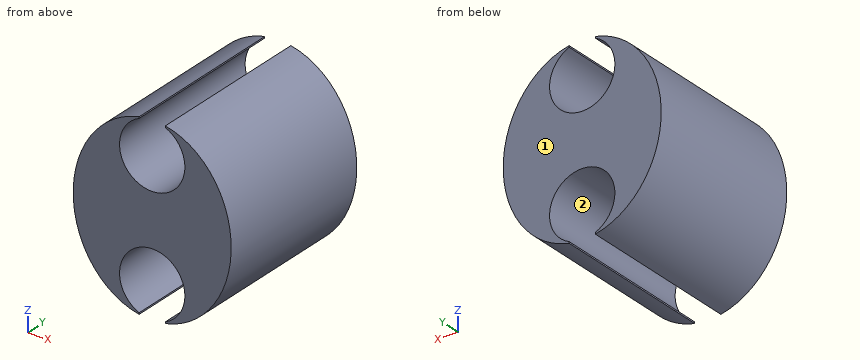
Autodesk Inventor part; units mm, degrees
ref_plane "YZ Plane" through (0, 0, 0) normal (1, 0, 0) x (0, 1, 0)
ref_plane "XZ Plane" through (0, 0, 0) normal (0, 1, 0) x (-1, 0, 0)
ref_plane "XY Plane" through (0, 0, 0) normal (0, 0, 1) x (1, 0, 0)
sketch "Boceto1" plane through (0, 0, 0) normal (0, 1, 0) x (-1, 0, 0)
  ellipse E0 centre (0, 0) end of major axis (0, 7) minor radius 6.05
  circle A0 centre (0, -4.5) radius 2.5
  circle A1 centre (0, 4.5) radius 2.5
  point P0 (0, 7)
  point P1 (0, -7)
  dimension "d0" = 7
  dimension "d1" = 6.05
  dimension "d6" = 5
  dimension "d7" = 5
extrude "Extrusión1" add sketch "Boceto1" along normal blind 13
sketch "Boceto2" plane through (0, 13, 4.5) normal (0, 1, 0) x (1, 0, 0)
  line L0 (-1, -2) -> (1, -2)
  line L1 (1, -2) -> (1, -4)
  line L2 (1, -4) -> (-1, -4)
  line L3 (-1, -4) -> (-1, -2)
  circle A0 centre (0, 0) radius 2.5
  point P0 (0, 4.5)
  point P1 (0, -2.5)
  dimension "d8" = 2
  dimension "d9" = 1
  dimension "d11" = 2
  dimension "d12" = 2
extrude "Extrusión2" cut sketch "Boceto2" against normal blind 13 contours L0 L1 A0 L3 | A0 L1 L2 L3 picked at (0, -2.1667)
sketch "Boceto4" plane through (0, 13, 0) normal (0, 1, 0) x (1, 0, 0)
  line L0 (-1, 8) -> (1, 8)
  line L1 (1, 8) -> (1, 4.3137)
  line L2 (1, 4.3137) -> (-1, 4.3137)
  line L3 (-1, 4.3137) -> (-1, 8)
  point P0 (0, 0)
  dimension "d15" = 2
  dimension "d16" = 4.3137
  dimension "d17" = 8
  dimension "d18" = 1
extrude "Extrusión3" cut sketch "Boceto4" against normal blind 13
equation "\"d7\" = d6"
properties part number "Relleno_chumacera" material "Plástico PC/ABS"
Geometry: final body of the model. Coordinates: model frame, mm. Face numbers are marked on the shaded views. Coordinates: 2 decimals unless noted, no trailing zeros. Order: outer loops, then holes, each group sorted by start corner. A loop starts at its lowest first (then second) coordinate and runs counter-clockwise, first axis right, second up. Notation, with made-up numbers: (20.5, 22) - (37.5, 22) arc R16 ccw to (37.5, 49) - close; hole circle Ø6 at (37.25, 5.5). An arc over 180 degrees is marked (long way). Return JSON: item names as keys, results as strings. Group by question number.
1. Cut plane A-A (x = 0). Output: boundary loops of the cut face in (y, z).
2. Pull-direction query (Z, two-part tool) for the marked faces 1 and 2; classes: pulls with the +Z half, pulls with the -Z half, needs draft (parallel to the pull), parting line crosses it, or undercut.
3. Material intervals for line 1 along Z through (x, y) = (0, 6.5); line 2 along X through (y, z) = (10, 5); line 3 along X through (y, z) = (6, 4.5), sorted ascending. Write a range as [from, to].
4. Pin query (flat end, axial travel): pin 1 (6 mm diameter, centred on y = 6.5, z = 4.5, fed in from +X); pin 2 (4.5 mm diameter, centred on x = 0, z = -4.5, fed in from -Y). Return the tip coordinate at first contact, or that it passes through.
5. Cut plane B-B (x = -1.5). Count the separate pieces of the cut face and the enclosed holes in it, plus the area to 3 significant figures.
Resolved:
{
 "1": {"outline": "(0, -2) - (13, -2) - (13, 2) - (0, 2) - close"},
 "2": {"face 1": "needs draft", "face 2": "undercut"},
 "3": {"line 1": "z = [-2, 2]", "line 2": "x = [-4.23, -2.45], [2.45, 4.23]", "line 3": "x = [-4.63, -2.5], [2.5, 4.63]"},
 "4": {"pin 1": "stops at x = 5.91", "pin 2": "passes through"},
 "5": {"separate pieces": "3", "enclosed holes": "0", "area": "72.3 mm²"}
}
